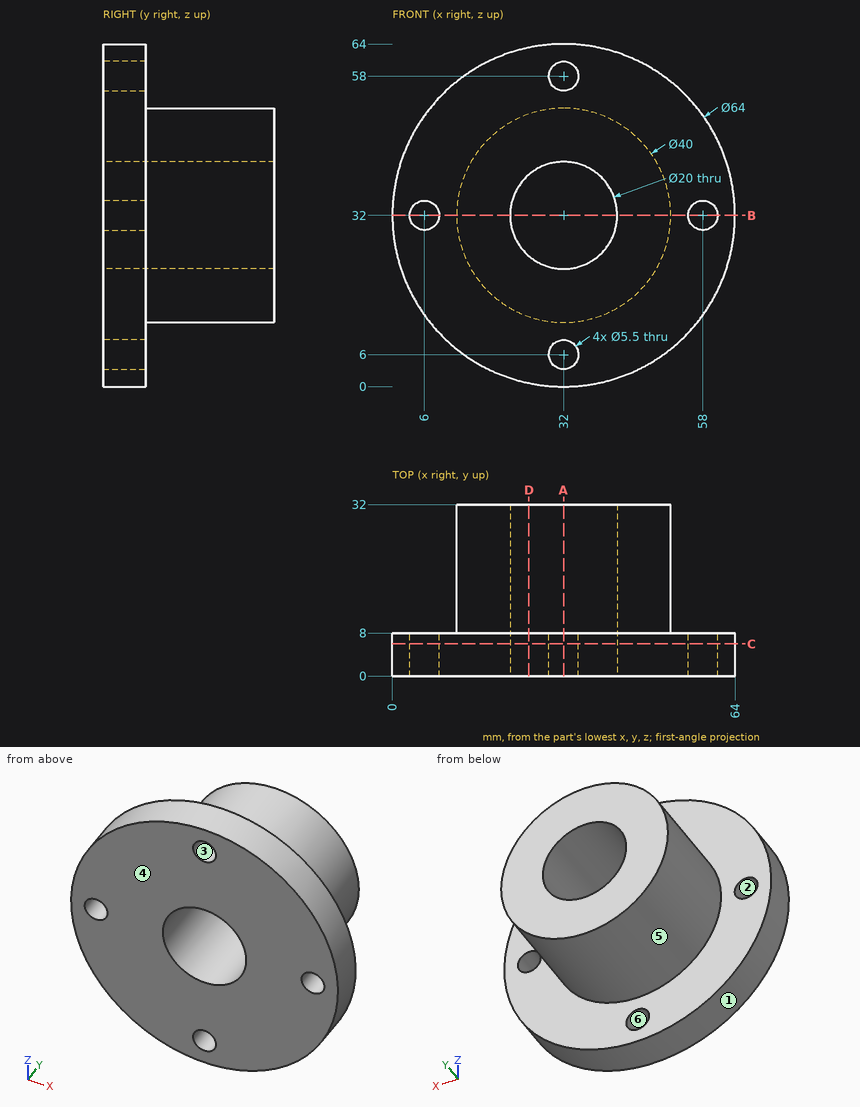
Could you check a few things on this drawing? It's one solid part, dimensions in mm from its lowest x, y, z. A direction names the side the tool comes from. Round coordinates to 2 decimals unless told otherwise and drop trailing zeros. Write each loop counter-clockwise with the first axis right and the second up, starting at its lowest first coordinate (ties: lowest second). Pieces come first, ordered by that corner, then holes. Notation, with made-up numbers: (84.25, 43) -> (98.25, 43) arc R21 cw to (98.25, 72) -> close; hole circle Ø3 at (44, -18.75). An arc over 180 degrees is marked (long way). One line per item, written item: value.
1) For the marked faces 5 and 6, which set-ups out of +Z, -Z, +X, -X, +Y, -Y let a thin tool reach every point of the face, with its end or its side?
Filled sheet:
face 5: +Y
face 6: +Y, -Y
2) We'd pull the mould along X, two halves only. Please class the marked faces 1, 2, 3 and 4: released by +X, released by -X, zero draft, split by the parting line, or undercut.
Filled sheet:
face 1: split by the parting line
face 2: undercut
face 3: undercut
face 4: zero draft
3) If I drill on line 1 (X direction, y = 4, z = 32); line 2 (X direction, y = 11, z = 32); line 3 (Y direction, x = 9, z = 50), over which ranges is the centre line in solid material (lowest first)? Write a range as [from, to].
Filled sheet:
line 1: x = [0, 3.25], [8.75, 22], [42, 55.25], [60.75, 64]
line 2: x = [12, 22], [42, 52]
line 3: y = [0, 8]
4) Suppose I cut it at B-B on z = 32. List the corners of the cut face in (x, y) for me, plus the area to 3 significant figures.
Filled sheet:
outline: (0, 0) -> (3.25, 0) -> (3.25, 8) -> (0, 8) -> close; (8.75, 0) -> (22, 0) -> (22, 32) -> (12, 32) -> (12, 8) -> (8.75, 8) -> close; (42, 0) -> (55.25, 0) -> (55.25, 8) -> (52, 8) -> (52, 32) -> (42, 32) -> close; (60.75, 0) -> (64, 0) -> (64, 8) -> (60.75, 8) -> close
area: 744 mm2
5) I'm going to push flat-ended pins straight in: pin 1 Ø5 at (x, z) = (32, 6) entering from -Y; pin 2 Ø3 at (y, z) = (25.5, 31.5) entering from +X; pin 3 Ø2 at (y, z) = (17.5, 22.5) entering from -X; pin 4 Ø8 at (x, z) = (18, 56) entering from +Y. Where does each tip first touch, or does it pass through?
Filled sheet:
pin 1: passes through
pin 2: stops at x = 52
pin 3: stops at x = 13.9
pin 4: stops at y = 8
6) Suppose I cut it at A-A on x = 32. List the corners of the cut face in (y, z) for me.
Filled sheet:
outline: (0, 0) -> (8, 0) -> (8, 3.25) -> (0, 3.25) -> close; (0, 8.75) -> (8, 8.75) -> (8, 12) -> (32, 12) -> (32, 22) -> (0, 22) -> close; (0, 42) -> (32, 42) -> (32, 52) -> (8, 52) -> (8, 55.25) -> (0, 55.25) -> close; (0, 60.75) -> (8, 60.75) -> (8, 64) -> (0, 64) -> close
7) Suppose I cut it at C-C on y = 6. List the corners of the cut face in (x, z) for me, plus the area to 3 significant figures.
Filled sheet:
outline: circle Ø64 at (32, 32); hole circle Ø5.5 at (6, 32); hole circle Ø20 at (32, 32); hole circle Ø5.5 at (32, 6); hole circle Ø5.5 at (32, 58); hole circle Ø5.5 at (58, 32)
area: 2,810 mm2
8) Suppose I cut it at D-D on x = 25.5. List the corners of the cut face in (y, z) for me, plus the area to 3 significant figures.
Filled sheet:
outline: (0, 0.67) -> (8, 0.67) -> (8, 13.09) -> (32, 13.09) -> (32, 24.4) -> (0, 24.4) -> close; (0, 39.6) -> (32, 39.6) -> (32, 50.91) -> (8, 50.91) -> (8, 63.33) -> (0, 63.33) -> close
area: 923 mm2
